Geometry: final body of the model. Coordinates: model frame, mm. Round coordinates to 2 decimals unless told otherwise and drop trailing zeros. Write each loop counter-clockwise with the first axis right and the second up, starting at its lowest first coordinate (ties: lowest second). Pieces come first, ordered by that corner, then holes. Notation, with made-up numbers: M -3,86.25 L 27,86.25 A15 cw 27,115.25 Z; hole C 36,-31.75 d11. An arc over 180 degrees is marked long. Use one line per item in the form item = value. Start each with the question number.
Item 1: Section query D-D (x = -46). Return loops of the section in (y, z), and give its area (3 significant figures).
Item 2: Ray query, probe 1 along Y at (x, z) = (32, 38); probe 2 along Z at (x, y) = (-63.5, 1.95); probe 3 along X at (y, z) = (0.7, 72.5). Return the intervals inside material, ascending.
Item 3: Section query C-C (x = 8). Return loops of the section in (y, z).
Item 4: Section query B-B (y = 1.9). Return loops of the section in (x, z).
Item 5: Pin query (flat end, axial travel): pin 1 Ø1.5 at (x, z) = (-51, -2) entering from +Y; pin 2 Ø1 at (x, y) = (-58.5, 2) entering from +Z; pin 3 Ø0.8 at (x, y) = (-5, 3) entering from -Z. Return the tip coordinate at first contact, or that it passes through.
Item 6: Section query A-A (z = -17). Return loops of the section in (x, y), and give its area (3 significant figures).
from build123d import *

# Parameters (mm, degrees)
BOSS_EXTRUDE1_DEPTH = 2.5
SKETCH2_W           = 25
SKETCH2_H           = 70
BOSS_EXTRUDE2_DEPTH = 1


with BuildPart() as part:
    # Sketch1 → Boss-Extrude1 (new body)
    with BuildSketch(Plane(origin=(0, 0, 0), x_dir=(1, 0, 0), z_dir=(0, 1, 0))):
        Polygon((73.612159322, 42.5), (0, 85), (-73.612159322, 42.5), (-73.612159322, -42.5), (0, -85), (73.612159322, -42.5), align=None)
    extrude(amount=BOSS_EXTRUDE1_DEPTH)

    # Sketch2 → Boss-Extrude2 (add)
    with BuildSketch(Plane(origin=(0, 2.5, 0), x_dir=(1, 0, 0), z_dir=(0, 1, 0))):
        Rectangle(SKETCH2_W, SKETCH2_H)
    extrude(amount=BOSS_EXTRUDE2_DEPTH)


solid = part.part
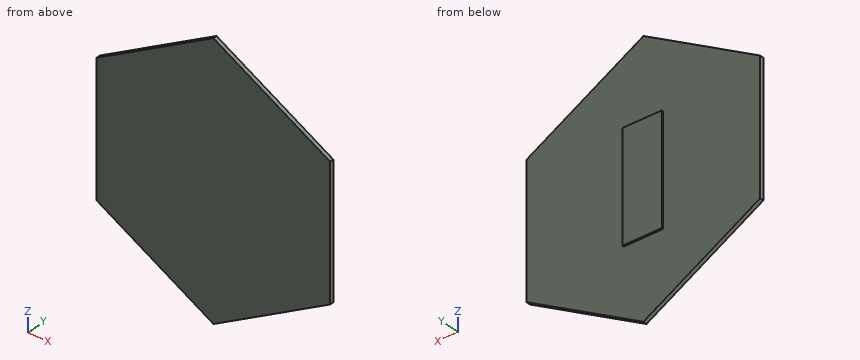
Working result:
q1.outline = M 0,-58.44 L 2.5,-58.44 L 2.5,58.44 L 0,58.44 Z
q1.area = 292 mm²
q2.probe_1 = 0 to 2.5
q2.probe_2 = -48.34 to 48.34
q2.probe_3 = -21.65 to 21.65
q3.outline = M 0,-80.38 L 2.5,-80.38 L 2.5,-35 L 3.5,-35 L 3.5,35 L 2.5,35 L 2.5,80.38 L 0,80.38 Z
q4.outline = M -73.61,-42.5 L 0,-85 L 73.61,-42.5 L 73.61,42.5 L 0,85 L -73.61,42.5 Z
q5.pin_1 = 2.5
q5.pin_2 = 51.51
q5.pin_3 = -35
q6.outline = M -73.61,0 L 73.61,0 L 73.61,2.5 L 12.5,2.5 L 12.5,3.5 L -12.5,3.5 L -12.5,2.5 L -73.61,2.5 Z
q6.area = 393 mm²
